from build123d import *

# Parameters (mm, degrees)
BOSS_EXTRUDE1_OUTLINE_R   = 1.5
BOSS_EXTRUDE1_OUTLINE_R_2 = 2.625
BOSS_EXTRUDE1_DEPTH       = 3.05


# Read off the part's stored shape, not the designer's step: Boss-Extrude1
with BuildPart() as part:
    # Boss-Extrude1 outline → Boss-Extrude1 (new body)
    with BuildSketch(Plane.XY):
        with BuildLine():
            ThreePointArc((-4.057068102, 31.544047144), (-5.473136356, 40.107888765), (-13.427731373, 36.633834833))
            add(Edge.make_bspline(
                [(-17.229515242, 31.01562696), (-14.514237852, 33.142129435), (-13.427731373, 36.633834833)],
                knots=[0, 0, 0, 1, 1, 1], degree=2))
            Line((-17.229515242, 31.01562696), (-19.754600441, 29.293942889))
            Line((-19.754600441, 29.293942889), (-17.9237303, 26.608721385))
            Line((-17.9237303, 26.608721385), (-13.932796466, 29.329868067))
            add(Edge.make_bspline(
                [(-13.932796466, 29.329868067), (-12.381551692, 30.407849096), (-10.691589638, 30.789278346), (-9.223592818, 29.609717336), (-7.813226831, 25.104795624)],
                knots=[0, 0, 0, 0, 0.517103648, 1, 1, 1, 1], degree=3))
            Line((-7.813226831, 25.104795624), (0, 0))
            Line((0, 0), (13, 0))
            Line((13, 0), (13, 6.303908615))
            Line((13, 6.303908615), (0.708529353, 16.231634907))
            Line((0.708529353, 16.231634907), (-4.057068102, 31.544047144))
        make_face()
        with Locations((3.4, 3.4)):
            Circle(BOSS_EXTRUDE1_OUTLINE_R, mode=Mode.SUBTRACT)
        Polygon((3.95568576, 11.322036253), (11.073847559, 5.572751724), (9.063168816, 3.083339947), (1.945007017, 8.832624477), align=None, mode=Mode.SUBTRACT)
        with Locations((-8.098279353, 35.2748127)):
            Circle(BOSS_EXTRUDE1_OUTLINE_R_2, mode=Mode.SUBTRACT)
    extrude(amount=BOSS_EXTRUDE1_DEPTH)

    # Sketch3 → CSK for M3 Flat Head Machine Screw1 (revolve, cut)
    with BuildSketch(Plane(origin=(3.4, 3.4, 3.05), x_dir=(0, -1, 0), z_dir=(1, 0, 0))):
        Polygon((0, 0), (0, 3.05), (1.55, 3.05), (1.55, 1.6), (3.15, 0), align=None)
    revolve(axis=Axis((3.4, 3.4, 9.4), (0, 0, -1)), mode=Mode.SUBTRACT)


solid = part.part
Build history of the part. All positions in model axes, mm. A direction names the side the tool comes from. Round coordinates to 2 decimals unless told otherwise and drop trailing zeros. Write each loop counter-clockwise with the first axis right and the second up, starting at its lowest first coordinate (ties: lowest second). Pieces come first, ordered by that corner, then holes. Notation, with made-up numbers: M 88,59.5 L 141,59.5 A19 cw 141,84.5 Z; hole C -34,58.25 d8. An arc over 180 degrees is marked long. Answer as a JSON object with one key per item and string values. Group by question number.
(1) Cut at B-B (x = 3.4). Give the cut face in (y, z).
(2) Cut at A-A (x = -6.5). Give the cut face in (y, z).
(3) Cut at C-C (y = 4.5). Give the number of separate pieces and of enclosed holes in the cut face, and give its area (3 significant figures).
(4) Mould opens along Y. For faces 1 (the flat face through (-3, 22, 3.05)), 2 (the flat face through (-18.47, 30.17, 1.5)), 3 (the cylindrical face through (-8.667, 32.712, 1.504)) say: pulls with the +Y half, pulls with the -Y half, needs draft (parallel to the pull), parting line crosses it, or undercut.
(5) Drill centre lines: L1, parallel to X at y = 3.4, z = 0.7; L2, parallel to Y at x = 4, z = 2.85; L3, parallel to Y at x = 2.5, z = 1.95. Where is each one in solid material? Low to high.
(6) Which spindle directions (+Z, -Z, +X, -X, +Y, -Y) get a long thin tool onto all of the face, cutting with end or side? Do faces 4 (the flat face through (-15.96, 27.95, 1.5)), 5 (the flat face through (10.083, 4.345, 1.504)), 6 (the flat face through (-1.64, 23.78, 1.5)). Say none if no direction does.
(7) Flat gauge pins, fed straight in: pin 1 (4.5 mm diameter, centred on x = -8.1, y = 35.27, fed in from -Z); pin 2 (5 mm diameter, centred on x = 3.4, y = 3.4, fed in from -Z). Where does each tip first touch, or does it go through?
Responses:
{
 "1": {"outline": "M 0,0 L 1.85,0 L 1.85,1.45 L 0.25,3.05 L 0,3.05 Z; M 4.95,0 L 7.66,0 L 7.66,3.05 L 6.55,3.05 L 4.95,1.45 Z; M 10.63,0 L 14.06,0 L 14.06,3.05 L 10.63,3.05 Z"},
 "2": {"outline": "M 20.89,0 L 33.19,0 L 33.19,3.05 L 20.89,3.05 Z; M 37.36,0 L 40.54,0 L 40.54,3.05 L 37.36,3.05 Z"},
 "3": {"separate pieces": "3", "enclosed holes": "0", "area": "25.3 mm2"},
 "4": {"face 1": "needs draft", "face 2": "pulls with the +Y half", "face 3": "undercut"},
 "5": {"L1": "x = -1.06 to 1.85, 4.95 to 8.67, 9.32 to 13", "L2": "y = 0 to 0.51, 6.29 to 7.17, 11.29 to 13.57", "L3": "y = 0 to 1.56, 5.24 to 8.38, 9.52 to 14.78"},
 "6": {"face 4": "+Z, -Z, -Y", "face 5": "+Z, -Z", "face 6": "+Z, -Z, +X"},
 "7": {"pin 1": "passes through", "pin 2": "stops at z = 0"}
}
